Autodesk Inventor part; units mm, degrees
ref_plane "Work Plane1" through (29, 0, 0) normal (0, -1, 0) x (1, 0, 0)
ref_plane "YZ Plane" through (0, 0, 0) normal (1, 0, 0) x (0, 1, 0)
ref_plane "XZ Plane" through (0, 0, 0) normal (0, 1, 0) x (-1, 0, 0)
sketch "Sketch1" plane through (0, 0, 0) normal (0, 0, 1) x (1, 0, 0)
  line L0 (0.2879, 0) -> (12.7, 0)
  line L1 (12.7, 0) -> (12.7, 2.413)
  line L2 (12.7, 2.413) -> (2.1084, 2.413)
  line L3 (2.1084, 2.413) -> (0.0001, 2.413)
  line L4 (0.0001, 2.413) -> (0, 2.413)
  line L5 (0, 2.413) -> (0, 4.5847)
  line L6 (0, 4.5847) -> (-2.5654, 4.5847)
  line L7 (-2.5654, 4.5847) -> (-2.5654, 1.8624)
  line L8 (-2.5654, 1.8624) -> (-0.7874, 1.8624)
  line L9 (-0.7874, 1.8624) -> (0.2879, 0)
  line L10 (-5.6185, 0) -> (15.7531, 0)
  line L11 (0, -0.9169) -> (0, 5.5016)
  line L12 (2.1084, 2.413) -> (0, 2.413) construction
  dimension "d1" = 10.5916
  dimension "d2" = 2.1083
  dimension "d3" = 2.5654
  dimension "d4" = 1.778
  dimension "d5" = 60
  dimension "d6" = 4.826
  dimension "d7" = 4.826
  dimension "d8" = 3.7248
  dimension "d9" = 9.1694
  dimension "d26" = 12.7
revolve "Body" add sketch "Sketch1" angle 360 about axis through (0.2879, 0, 0) along (1, 0, 0) contours L9 L11 L3 L2 L1 L0 | L9 L8 L7 L6 L5 L11
sketch "Sketch2" plane through (-2.5654, 0, 0) normal (-1, 0, 0) x (0, 0, 1)
  circle A0 centre (0, 0) radius 1.8624
  line L0 (0, -6.4186) -> (0, 6.4186)
  line L1 (-6.4186, 0) -> (6.4186, 0)
  line L2 (1.8624, 0) -> (0.9312, -1.6129)
  line L3 (0.9312, -1.6129) -> (-0.9312, -1.6129)
  line L4 (-0.9312, -1.6129) -> (-1.8624, 0)
  line L5 (-1.8624, 0) -> (-0.9312, 1.6129)
  line L6 (-0.9312, 1.6129) -> (0.9312, 1.6129)
  line L7 (0.9312, 1.6129) -> (1.8624, 0)
extrude "Slot" add sketch "Sketch2" against normal up to next contours L7 A0 | A0 L2 | L6 L0 A0 | A0 L0 L3 | L0 L6 A0 | A0 L3 L0 | L4 A0 | A0 L5
fillet "Fillet1" radius 2.0574 1 edges at (-2.5654, -4.5847, 0)
thread "Thread"
chamfer "Chamfer1" distance 0.4724 distance2 0.4724 1 edges at (12.7, -2.413, 0) measured on face at (12.7, -0.2852, -0.7521)
ref_plane "Work Plane1" through (29, 0, 0) normal (0, -1, 0) x (1, 0, 0)
fillet "Fillet2" radius 0.1 1 edges at (0.0001, -2.413, 0)
equation "\"d30\" = R"
equation "\"d17\" = RR"
equation "\"d13\" = GEL"
equation "\"d15\" = -0.5 * SPD + 0.5 * GD"
equation "\"d16\" = GUL"
equation "\"d1\" = GEL"
equation "\"d3\" = KOH"
equation "\"d4\" = INTI"
equation "\"d6\" = GD"
equation "\"d7\" = BDM"
equation "\"d8\" = 1.1547 * SW"
equation "\"d9\" = KOD"
equation "\"d26\" = NLG"
equation "\"GD\" = NND"
equation "\"NLG\" = 12.7"
equation "\"GEL\" = 10.5916"
equation "\"KOD\" = 9.1694"
equation "\"KOH\" = 2.5654"
equation "\"INTI\" = 1.778"
equation "\"GAL\" = 2.1082"
equation "\"GUL\" = 0.47244"
equation "\"BDM\" = NND"
equation "\"SW\" = 3.2258"
equation "\"RR\" = 2.0574"
equation "\"SPD\" = 3.88112"
equation "\"R\" = 0.1"
equation "\"TOA\" = 30deg"
equation "\"GD1\" = SPD"
equation "\"THREADDIA\" = 4.826"
equation "\"KOH1\" = 0.508"
equation "\"NND\" = 4.826"
equation "\"E0\" = 3.72593"
properties part number "ANSI B18.3 - No. 10-32 - 1/2, HSBHCSI" material "Steel, Mild"
Design review of the part built by this model. Coordinates are the model's own, in mm. A direction names the side the tool comes from. Round coordinates to 2 decimals unless told otherwise and drop trailing zeros. Order: outer loops, then holes, each group sorted by start corner. A loop starts at its lowest first (then second) coordinate and runs counter-clockwise, first axis right, second up. Notation, with made-up numbers: (-2.5, -37) - (56.5, -37) arc R15 ccw to (56.5, -9) - close; hole circle Ø6 at (-33.5, 34.5). An arc over 180 degrees is marked (long way). One line per question, with ' | ' between items.
Item 1: For P1, Ø0.6, axis at x = -2, z = 0, coming from the +Y side; P2, Ø1, axis at x = 5, y = 0.5, coming from the -Z side; P3, Ø5, axis at x = 11, z = 3.5, coming from the -Y side; P4, Ø1.5, axis at x = 3.5, y = 3.5, coming from the -Z side, all flat-tipped, find the tip position at first contact; note any pin that passes through.
Checks:
P1: y = 4.2 | P2: z = -2.41 | P3: y = -2.2 | P4: through
Item 2: Wall thickness on line 1 (Y direction, x = 0.5, z = 0); line 2 (X direction, y = 1.5, z = 2); line 3 (X direction, y = 1, z = -2.75): over which ranges is each line inside the solid? List them lowest first. Write a range as [from, to].
Checks:
line 1: [-2.41, 2.41] | line 2: [-2.57, 0] | line 3: [-2.53, 0]
Item 3: Take a section at A-A, the plane x = 2.5. Write out the cut boundary in (y, z), then the cut area to 3 significant figures.
Checks:
outline: circle Ø4.83 at (0, 0) | area: 18.3 mm²
Item 4: Machinability: for faces 4 (the face through (-2, 1.613, 0)), 5 (the face through (0, -1, 3)), 6 (the face through (-0.26, -3.64, 2.79)), which of the approach directions +Z, -Z, +X, -X, +Y, -Y give a long, thin tool a straight path to every point of the face, cutting with its end or side? Answer none if there is none.
Checks:
face 4: -X | face 5: +X | face 6: +X, -X
Item 5: Draft analysis for pull direction Y (two halves, no side actions). For faces 1 (the face through (6.079, -1.915, 1.468)), 2 (the face through (12.7, 0, 0)), 3 (the face through (-1.6, 0.8, -1.4)), state which applies: +Y half, -Y half, draft (parallel to the pull), parting line (faces both ways), or undercut.
Checks:
face 1: parting line | face 2: draft | face 3: undercut
